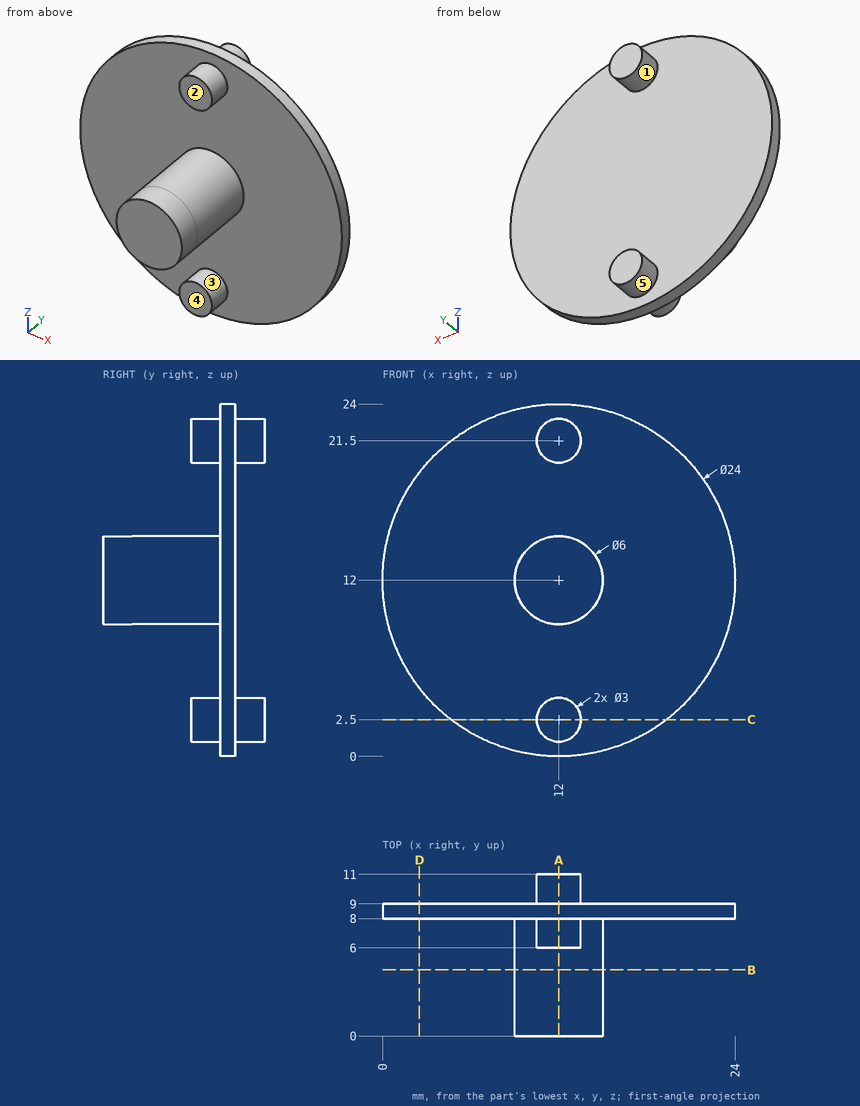
Check sheet for the drawn part. Datum: minimum x, y, z corner. Units: mm. A direction names the side the tool comes from. Coordinates: 2 decimals unless noted, no trailing zeros. Order: outer loops, then holes, each group sorted by start corner. A loop starts at its lowest first (then second) coordinate and runs counter-clockwise, first axis right, second up. Notation, with made-up numbers: M 43.25,88 L 101.25,88 A32 ccw 101.25,125 Z; hole C 59,-36 d10. An arc over 180 degrees is marked long. One line per item, written item: value. Start each with the question number.
Item 1: Gauge pin test, flat ends, axial feed: pin 1 (4 mm diameter, centred on x = 4.5, y = 5.5, fed in from -Z); pin 2 (1.5 mm diameter, centred on x = 16, z = 6, fed in from +Y); pin 3 (10 mm diameter, centred on x = 3, z = 19.5, fed in from -Y); pin 4 (2.5 mm diameter, centred on x = 12.5, z = 22, fed in from -Y). Record the tip position at first contact, or that the pin passes through.
Item 2: Mould release check, pull along Z, two halves, no side actions. Record for the marked faces 1 and 2: released by +Z, released by -Z, zero draft, split by the parting line, or undercut.
Item 3: Sectioned sample at B-B (y = 4.5). Enter the section's corners in (x, z), then the cut area to 3 significant figures.
Item 4: Sectioned sample at A-A (x = 12). Enter the section's corners in (y, z).
Item 5: Sectioned sample at C-C (z = 2.5). Enter the section's corners in (x, y), then the cut area to 3 significant figures.
Item 6: Scan lines: probe 1 along Z at (x, y) = (11.25, 7); probe 2 along Y at (x, z) = (15.25, 18.5); probe 3 along Y at (x, z) = (13, 21.75). Record each from-to range of solid material in increasing order.
Item 7: Access from +Z, -Z, +X, -X, +Y, -Y to the whole of each face (thin tool, end or side, straight path). Record for the marked faces 3, 4 and 5.
Item 8: Sectioned sample at D-D (x = 2.5). Enter the section's corners in (y, z), then the cut area to 3 significant figures.
Conclusion:
1. pin 1: passes through
1. pin 2: stops at y = 9
1. pin 3: stops at y = 8
1. pin 4: stops at y = 6
2. face 1: undercut
2. face 2: zero draft
3. outline: C 12,12 d6
3. area: 28.3 mm^2
4. outline: M 0,9 L 8,9 L 8,4 L 6,4 L 6,1 L 8,1 L 8,0 L 9,0 L 9,1 L 11,1 L 11,4 L 9,4 L 9,20 L 11,20 L 11,23 L 9,23 L 9,24 L 8,24 L 8,23 L 6,23 L 6,20 L 8,20 L 8,15 L 0,15 Z
5. outline: M 4.67,8 L 10.5,8 L 10.5,6 L 13.5,6 L 13.5,8 L 19.33,8 L 19.33,9 L 13.5,9 L 13.5,11 L 10.5,11 L 10.5,9 L 4.67,9 Z
5. area: 26.7 mm^2
6. probe 1: z = 1.2 to 3.8, 9.1 to 14.9, 20.2 to 22.8
6. probe 2: y = 8 to 9
6. probe 3: y = 6 to 11
7. face 3: -Y
7. face 4: -Z, +X, -X, -Y
7. face 5: +Y
8. outline: M 8,4.67 L 9,4.67 L 9,19.33 L 8,19.33 Z
8. area: 14.7 mm^2
